The listing builds one solid part. Answer for the finished solid, in the listing's coordinates (mm). Coordinates: 2 decimals unless noted, no trailing zeros. Order: outer loops, then holes, each group sorted by start corner. A loop starts at its lowest first (then second) coordinate and runs counter-clockwise, first axis right, second up. Notation, with made-up numbers: (-7, 11.25) -> (23, 11.25) arc R21 ccw to (23, 43.25) -> close; hole circle Ø2 at (52, -31). An arc over 180 degrees is marked (long way). Answer in a Markdown table with one row per item.
```python
from build123d import *

# Parameters (mm, degrees)
SKETCH_1_R      = 15
SKETCH_1_R_2    = 20
SKETCH_1_R_3    = 22.5
EXTRUDE_1_DEPTH = 4


with BuildPart() as part:
    # 草图1 → 凸台-拉伸1 (new body)
    with BuildSketch(Plane.XY):
        with BuildLine():
            Line((-315.638914213, 504.066678813), (-315.638914213, 430.95617818))
            Line((-315.638914213, 430.95617818), (84.361085787, 430.95617818))
            Line((84.361085787, 430.95617818), (84.361085787, 504.066678813))
            ThreePointArc((84.361085787, 504.066678813), (82.42300747, 509.287129513), (77.547809411, 511.978169636))
            Line((77.547809411, 511.978169636), (-103.638914213, 539.15617818))
            Line((-103.638914213, 539.15617818), (-103.638914213, 537.15617818))
            Line((-103.638914213, 537.15617818), (-127.638914213, 537.15617818))
            Line((-127.638914213, 537.15617818), (-127.638914213, 539.15617818))
            Line((-127.638914213, 539.15617818), (-308.825637836, 511.978169636))
            ThreePointArc((-308.825637836, 511.978169636), (-313.700835896, 509.287129513), (-315.638914213, 504.066678813))
        make_face()
        with Locations((50.361085787, 480.95617818)):
            Circle(SKETCH_1_R, mode=Mode.SUBTRACT)
        with Locations((-5.638914213, 488.45617818)):
            Circle(SKETCH_1_R_2, mode=Mode.SUBTRACT)
        with Locations((-70.638914213, 492.20617818)):
            Circle(SKETCH_1_R_3, mode=Mode.SUBTRACT)
        with Locations((-281.638914213, 480.95617818)):
            Circle(SKETCH_1_R, mode=Mode.SUBTRACT)
        with Locations((-225.638914213, 488.45617818)):
            Circle(SKETCH_1_R_2, mode=Mode.SUBTRACT)
        with Locations((-160.638914213, 492.20617818)):
            Circle(SKETCH_1_R_3, mode=Mode.SUBTRACT)
    extrude(amount=EXTRUDE_1_DEPTH)


solid = part.part
```
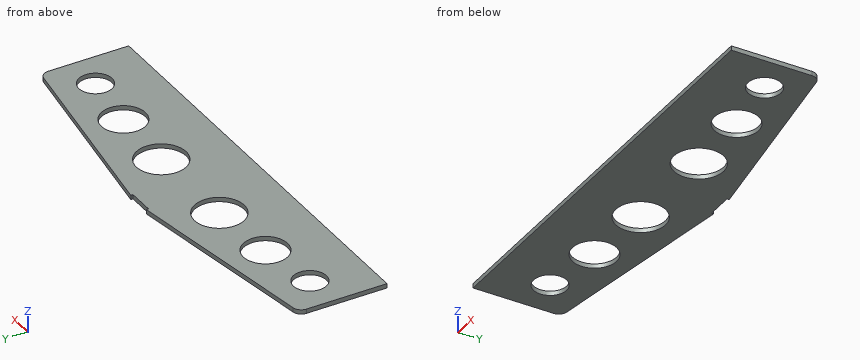
(1) A cutting plane is placed at D-D, the plane y = 522. Determine the outline of the cut face in (x, z).
Check values:
| item | result |
|---|---|
| outline | (-242.01, 0) -> (10.74, 0) -> (10.74, 4) -> (-242.01, 4) -> close |
(2) A cutting plane is placed at C-C, the plane x = -167.5. Determine the outline of the cut face in (y, z), then the cut area to 3 significant figures.
Check values:
| item | result |
|---|---|
| outline | (430.96, 0) -> (470.78, 0) -> (470.78, 4) -> (430.96, 4) -> close; (513.63, 0) -> (533.18, 0) -> (533.18, 4) -> (513.63, 4) -> close |
| area | 237 mm² |
(3) A cutting plane is placed at A-A, the plane z = 0.6. Determine the outline of the cut face in (x, y), then the cut area to 3 significant figures.
Check values:
| item | result |
|---|---|
| outline | (-315.64, 430.96) -> (84.36, 430.96) -> (84.36, 504.07) arc R8 ccw to (77.55, 511.98) -> (-103.64, 539.16) -> (-103.64, 537.16) -> (-127.64, 537.16) -> (-127.64, 539.16) -> (-308.83, 511.98) arc R8 ccw to (-315.64, 504.07) -> close; hole circle Ø30 at (-281.64, 480.96); hole circle Ø40 at (-225.64, 488.46); hole circle Ø45 at (-160.64, 492.21); hole circle Ø45 at (-70.64, 492.21); hole circle Ø40 at (-5.64, 488.46); hole circle Ø30 at (50.36, 480.96) |
| area | 30,800 mm² |
(4) Find the intervals of material crossed by line 1 along X through (y, z) = (510.5, 0.65); line 2 along Y through (x, z) = (-271, 1.55); line 3 along Y through (x, z) = (-147, 3.55), in increasing order. Write a range as from..to.
Check values:
| item | result |
|---|---|
| line 1 | -312.39..-173.74, -147.54..-83.74, -57.54..81.12 |
| line 2 | 430.96..470.38, 491.53..517.65 |
| line 3 | 430.96..474.31, 510.1..536.25 |
(5) A cutting plane is placed at B-B, the plane x = -60. Determine the outline of the cut face in (y, z).
Check values:
| item | result |
|---|---|
| outline | (430.96, 0) -> (472.38, 0) -> (472.38, 4) -> (430.96, 4) -> close; (512.03, 0) -> (532.61, 0) -> (532.61, 4) -> (512.03, 4) -> close |
